from build123d import *

# Parameters (mm, degrees)
F1_DEPTH = 8
F2_R     = 0.5
F3_R     = 0.2


with BuildPart() as f1:
    # F0 (on Top) → F1 (new body)
    with BuildSketch(Plane.XY):
        Polygon((0, 8.6), (0, 0), (0.8, 0), (0.8, 6.8), (0.8, 8.6), align=None)
        Polygon((0.8, 0), (0, 0), (0, -0.8), (22.2, -0.8), (22.2, 0), (21.4, 0), align=None)
        Polygon((21.4, 6.8), (21.4, 0), (22.2, 0), (22.2, 8.6), (21.4, 8.6), align=None)
        with BuildLine():
            ThreePointArc((19.4, 6.8), (20.4, 7.3), (21.4, 6.8))
            Line((21.4, 6.8), (21.4, 8.6))
            Line((21.4, 8.6), (19.4, 8.6))
            Line((19.4, 8.6), (19.4, 6.8))
        make_face()
        with BuildLine():
            Line((0.8, 8.6), (0.8, 6.8))
            ThreePointArc((0.8, 6.8), (1.8, 7.3), (2.8, 6.8))
            Line((2.8, 6.8), (2.8, 8.6))
            Line((2.8, 8.6), (0.8, 8.6))
        make_face()
    extrude(amount=F1_DEPTH)

    # F2
    f2_edges = [f1.edges().sort_by_distance(p)[0] for p in [
        (22.2, -0.8, 4),
        (0, -0.8, 4),
        (22.2, 8.6, 4),
        (19.4, 8.6, 4),
        (0, 8.6, 4),
        (2.8, 8.6, 4),
        (0.8, 0, 4),
        (21.4, 0, 4),
    ]]
    fillet(f2_edges, radius=F2_R)

    # F3
    f3_edges = [f1.edges().sort_by_distance(p)[0] for p in [
        (2.8, 6.8, 4),
        (0.8, 6.8, 4),
        (19.4, 6.8, 4),
        (21.4, 6.8, 4),
    ]]
    fillet(f3_edges, radius=F3_R)


solid = f1.part
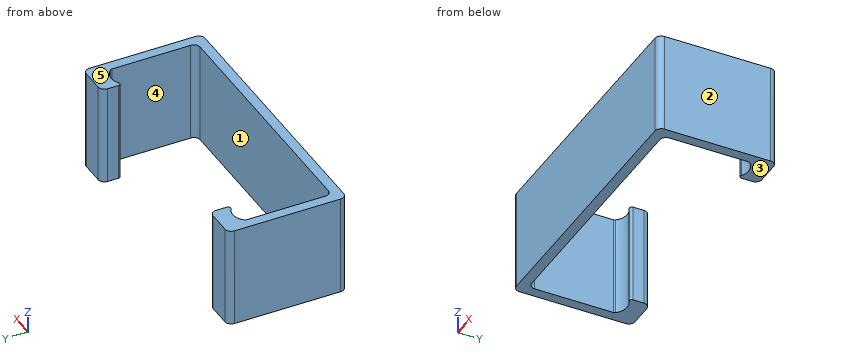
The listing builds one solid part. Answer for the finished solid, in the listing's coordinates (mm). Face numbers are marked on the shaded views. A direction names the side the tool comes from. Round coordinates to 2 decimals unless told otherwise and drop trailing zeros. Write each loop counter-clockwise with the first axis right and the second up, starting at its lowest first coordinate (ties: lowest second). Pieces come first, ordered by that corner, then holes. Notation, with made-up numbers: (47.25, -36.75) - (69.25, -36.75) arc R15 cw to (69.25, -19.75) - close; hole circle Ø9 at (-22.75, 85). An arc over 180 degrees is marked (long way). Use a Markdown table: item, result. Add a question column.
1. The part is cut by section B-B (x = 20.25). Write down the section's boundary in (y, z), and give its area (3 significant figures).
2. For a pull along X with two mould halves and no side action, classify the marked faces 1, 2 and 3 as +X half, -X half, draft (parallel to the pull), parting line (faces both ways), or undercut.
3. The part is cut by section C-C (z = 2.5). Write down the section's boundary in (x, y).
4. The part is cut by section A-A (y = 3.75). Write down the section's boundary in (x, z).
5. A flat-ended cylindrical pin translates along its axis: P1, Ø4, axis at x = 15, z = 2, coming from the +Y side. Find the tip coordinate at first contact, or state that the pin passes through.
6. The part is cut by section D-D (x = 17.25). Write down the section's boundary in (y, z).
7. Consider line 1 (X direction, y = 6, z = 4); line 2 (X direction, y = 8, z = 2); line 3 (Y direction, x = 3.75, z = 2). Determine where each line is inside the solid, lowest interval first.
8. A tool of negligible diameter and unlimited length cuts with its end or side. For the marked faces 4 and 5, from which of +Z, -Z, +X, -X, +Y, -Y can it reach the whole face along a straight path? Write none if from no direction.
Reported:
| question | item | result |
|---|---|---|
| 1 | outline | (-0.8, 0) - (0, 0) - (0, 8) - (-0.8, 8) - close; (7.29, 0) - (8.6, 0) - (8.6, 8) - (7.29, 8) - close |
| 1 | area | 16.9 mm^2 |
| 2 | face 1 | undercut |
| 2 | face 2 | +X half |
| 2 | face 3 | draft |
| 3 | outline | (0, -0.3) arc R0.5 ccw to (0.5, -0.8) - (21.7, -0.8) arc R0.5 ccw to (22.2, -0.3) - (22.2, 8.1) arc R0.5 ccw to (21.7, 8.6) - (19.9, 8.6) arc R0.5 ccw to (19.4, 8.1) - (19.4, 7.26) arc R0.2 ccw to (19.71, 7.09) arc R1.25 cw to (21.35, 6.86) arc R0.2 cw to (21.4, 6.73) - (21.4, 0.5) arc R0.5 cw to (20.9, 0) - (1.3, 0) arc R0.5 cw to (0.8, 0.5) - (0.8, 6.73) arc R0.2 cw to (0.85, 6.86) arc R1.25 cw to (2.49, 7.09) arc R0.2 ccw to (2.8, 7.26) - (2.8, 8.1) arc R0.5 ccw to (2.3, 8.6) - (0.5, 8.6) arc R0.5 ccw to (0, 8.1) - close |
| 4 | outline | (0, 0) - (0.8, 0) - (0.8, 8) - (0, 8) - close; (21.4, 0) - (22.2, 0) - (22.2, 8) - (21.4, 8) - close |
| 5 | P1 | y = 0 |
| 6 | outline | (-0.8, 0) - (0, 0) - (0, 8) - (-0.8, 8) - close |
| 7 | line 1 | 0 to 0.8, 21.4 to 22.2 |
| 7 | line 2 | 0 to 2.8, 19.4 to 22.2 |
| 7 | line 3 | -0.8 to 0 |
| 8 | face 4 | +Z, -Z |
| 8 | face 5 | +Z, +X, -X, +Y, -Y |
